CAD build for the part. Positions are in the model's coordinates, mm. Face numbers are marked on the shaded views. A direction names the side the tool comes from. Give positions to 0.01 mm unless a question says otherwise; leave off trailing zeros. Write each loop counter-clockwise with the first axis right and the second up, starting at its lowest first coordinate (ties: lowest second). Pieces come first, ordered by that corner, then holes. Notation, with made-up numbers: (17, -2) -> (69, -2) arc R13 cw to (69, 10) -> close; hole circle Ø8 at (80.5, 53). An arc over 180 degrees is marked (long way). Answer as a JSON object with one key per item and string values.
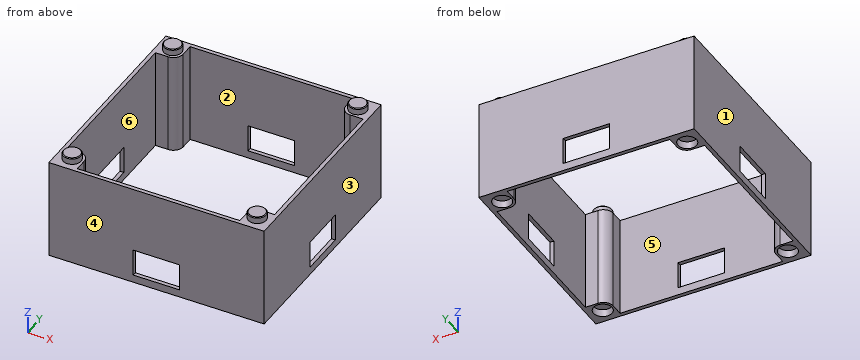
```python
from build123d import *

# Parameters (mm, degrees)
SKICA1_W                 = 5.8
SKICA1_H                 = 5.8
SKICA1_W_2               = 1
SKICA1_H_2               = 42
SKICA1_W_3               = 42
SKICA1_H_3               = 1
P_IDAT_VYSUNUT_M2_DEPTH  = 26
ZAOBLIT1_R               = 2.5
SKICA2_R                 = 2.4
ODEBRAT_VYSUNUT_M1_DEPTH = 1.9
SKICA3_R                 = 2.3
P_IDAT_VYSUNUT_M3_DEPTH  = 1.7
ZKOSEN_1_SIZE            = 0.2
SKICA4_W                 = 12
SKICA4_H                 = 7
ODEBRAT_VYSUNUT_M2_DEPTH = 68.7
SKICA5_W                 = 7
SKICA5_H                 = 12
ODEBRAT_VYSUNUT_M3_DEPTH = 55.6


with BuildPart() as part:
    # Skica1 → Přidat vysunutím2 (new body)
    with BuildSketch(Plane.XY):
        Polygon((-27.8, 27.8), (-27.8, 21), (-26.8, 21), (-26.8, 26.8), (-21, 26.8), (-21, 27.8), align=None)
        with Locations((-23.9, 23.9)):
            Rectangle(SKICA1_W, SKICA1_H)
        Polygon((26.8, 21), (27.8, 21), (27.8, 27.8), (21, 27.8), (21, 26.8), (26.8, 26.8), align=None)
        with Locations((23.9, 23.9)):
            Rectangle(SKICA1_W, SKICA1_H)
        Polygon((21, -26.8), (21, -27.8), (27.8, -27.8), (27.8, -21), (26.8, -21), (26.8, -26.8), align=None)
        with Locations((23.9, -23.9)):
            Rectangle(SKICA1_W, SKICA1_H)
        with Locations((-23.9, -23.9)):
            Rectangle(SKICA1_W, SKICA1_H)
        Polygon((-27.8, -27.8), (-21, -27.8), (-21, -26.8), (-26.8, -26.8), (-26.8, -21), (-27.8, -21), align=None)
        with Locations((-27.3, 0)):
            Rectangle(SKICA1_W_2, SKICA1_H_2)
        with Locations((0, -27.3)):
            Rectangle(SKICA1_W_3, SKICA1_H_3)
        with Locations((27.3, 0)):
            Rectangle(SKICA1_W_2, SKICA1_H_2)
        with Locations((0, 27.3)):
            Rectangle(SKICA1_W_3, SKICA1_H_3)
    extrude(amount=P_IDAT_VYSUNUT_M2_DEPTH)

    # Zaoblit1
    zaoblit1_edges = [part.edges().sort_by_distance(p)[0] for p in [
        (21, -21, 13),
        (21, 21, 13),
        (-21, 21, 13),
        (-21, -21, 13),
    ]]
    fillet(zaoblit1_edges, radius=ZAOBLIT1_R)

    # Skica2 → Odebrat vysunutím1 (cut)
    with BuildSketch(Plane(origin=(0, 0, 0), x_dir=(-1, 0, 0), z_dir=(0, 0, -1))):
        with Locations((-23.9, 23.9)):
            Circle(SKICA2_R)
        with Locations((23.9, 23.9)):
            Circle(SKICA2_R)
        with Locations((23.9, -23.9)):
            Circle(SKICA2_R)
        with Locations((-23.9, -23.9)):
            Circle(SKICA2_R)
    extrude(amount=-ODEBRAT_VYSUNUT_M1_DEPTH, mode=Mode.SUBTRACT)

    # Skica3 → Přidat vysunutím3 (add)
    with BuildSketch(Plane.XY.offset(26)):
        with Locations((-23.9, 23.9)):
            Circle(SKICA3_R)
        with Locations((23.9, 23.9)):
            Circle(SKICA3_R)
        with Locations((23.9, -23.9)):
            Circle(SKICA3_R)
        with Locations((-23.9, -23.9)):
            Circle(SKICA3_R)
    extrude(amount=P_IDAT_VYSUNUT_M3_DEPTH)

    # Zkosení1
    zkosen_1_edges = [part.edges().sort_by_distance(p)[0] for p in [
        (-26.2, 23.9, 27.7),
        (21.6, 23.9, 27.7),
        (21.6, -23.9, 27.7),
        (-26.2, -23.9, 27.7),
    ]]
    chamfer(zkosen_1_edges, length=ZKOSEN_1_SIZE)

    # Skica4 → Odebrat vysunutím2 (cut)
    with BuildSketch(Plane(origin=(0, -27.8, 0), x_dir=(-1, 0, 0), z_dir=(0, -1, 0))):
        with Locations((0, -5.5)):
            Rectangle(SKICA4_W, SKICA4_H)
    extrude(amount=-ODEBRAT_VYSUNUT_M2_DEPTH, mode=Mode.SUBTRACT)

    # Skica5 → Odebrat vysunutím3 (cut)
    with BuildSketch(Plane.ZY.offset(27.8)):
        with Locations((5.5, 0)):
            Rectangle(SKICA5_W, SKICA5_H)
    extrude(amount=-ODEBRAT_VYSUNUT_M3_DEPTH, mode=Mode.SUBTRACT)


solid = part.part
```
1) Wall check: probe 1 along Y at (x, z) = (23.9, 1.3); probe 2 along Y at (x, z) = (8, 18.5). Give the ranges that are in metal, low to high.
Model answer:
{"probe 1": "y = -27.8 to -26.3, -21.5 to -21, 21 to 21.5, 26.3 to 27.8", "probe 2": "y = -27.8 to -26.8, 26.8 to 27.8"}
2) Slice it at A-A (y = -8). List the corners of the cut face in (x, z).
Model answer:
{"outline": "(-27.8, 0) -> (-26.8, 0) -> (-26.8, 26) -> (-27.8, 26) -> close; (26.8, 0) -> (27.8, 0) -> (27.8, 26) -> (26.8, 26) -> close"}
3) Slice it at D-D (x = -1). List the corners of the cut face in (y, z).
Model answer:
{"outline": "(-27.8, 0) -> (-26.8, 0) -> (-26.8, 2) -> (-27.8, 2) -> close; (-27.8, 9) -> (-26.8, 9) -> (-26.8, 26) -> (-27.8, 26) -> close; (26.8, 0) -> (27.8, 0) -> (27.8, 2) -> (26.8, 2) -> close; (26.8, 9) -> (27.8, 9) -> (27.8, 26) -> (26.8, 26) -> close"}
4) Mould opens along Y. For the marked faces 3, 4, 5 and 6 say: released by +Y, released by -Y, zero draft, split by the parting line, or undercut.
Model answer:
{"face 3": "zero draft", "face 4": "released by -Y", "face 5": "undercut", "face 6": "undercut"}
5) 3-axis set-ups, long thin cutter, end or side, ignore diameter. For the marked faces 1 and 2: which of +Z, -Z, +X, -X, +Y, -Y reach the whole face in a straight line?
Model answer:
{"face 1": "+Z, -Z, -X, +Y, -Y", "face 2": "+Z, -Z"}
6) Slice it at C-C (z = 10). List the corners of the cut face in (x, y), then the cut area to 3 significant figures.
Model answer:
{"outline": "(-27.8, -27.8) -> (27.8, -27.8) -> (27.8, 27.8) -> (-27.8, 27.8) -> close; hole (-26.8, -21) -> (-23.5, -21) arc R2.5 cw to (-21, -23.5) -> (-21, -26.8) -> (21, -26.8) -> (21, -23.5) arc R2.5 cw to (23.5, -21) -> (26.8, -21) -> (26.8, 21) -> (23.5, 21) arc R2.5 cw to (21, 23.5) -> (21, 26.8) -> (-21, 26.8) -> (-21, 23.5) arc R2.5 cw to (-23.5, 21) -> (-26.8, 21) -> close", "area": "348 mm2"}
7) Pin check, flat tips, straight feed: pin 1 (0.5 mm diameter, centred on x = -0.5, y = -27.5, fed in from +Z); pin 2 (1.4 mm diameter, centred on x = -24, y = -25, fed in from -Z). Stop position of each tip, or through.
Model answer:
{"pin 1": "stops at z = 26", "pin 2": "stops at z = 1.9"}
